Input: part model. Units: mm. Frame: model coordinates. Face numbers are marked on the shaded views. Coordinates: 2 decimals unless noted, no trailing zeros. Loops run counter-clockwise (first coordinate to the right, second up) from the corner with the lowest first, then second, coordinate; pieces in that order, holes last. Notation, with made-up numbers: (-15, 58) -> (43, 58) arc R30 cw to (43, 92) -> close; hole circle Ø4 at (-11.5, 48). An arc over 180 degrees is marked (long way). Answer as a JSON object with one key per item and string values.
from build123d import *

# Parameters (mm, degrees)
SKETCH_1_R          = 12.5
EXTRUDE_1_DEPTH     = 10
SKETCH_3_R          = 5
CUT_EXTRUDE_1_DEPTH = 11
CHAMFER_1_SIZE      = 7


with BuildPart() as part:
    # ｽｹｯﾁ1 → ﾎﾞｽ - 押し出し1 (new body)
    with BuildSketch(Plane.XY):
        Circle(SKETCH_1_R)
    extrude(amount=EXTRUDE_1_DEPTH)

    # ｽｹｯﾁ3 → ｶｯﾄ - 押し出し1 (cut, through all)
    with BuildSketch(Plane(origin=(0, 0, 0), x_dir=(-1, 0, 0), z_dir=(0, 0, -1))):
        Circle(SKETCH_3_R)
    extrude(amount=-CUT_EXTRUDE_1_DEPTH, mode=Mode.SUBTRACT)

    # 面取り1
    chamfer_1_edges = [part.edges().sort_by_distance(p)[0] for p in [
        (5, 0, 0),
    ]]
    chamfer(chamfer_1_edges, length=CHAMFER_1_SIZE)


solid = part.part
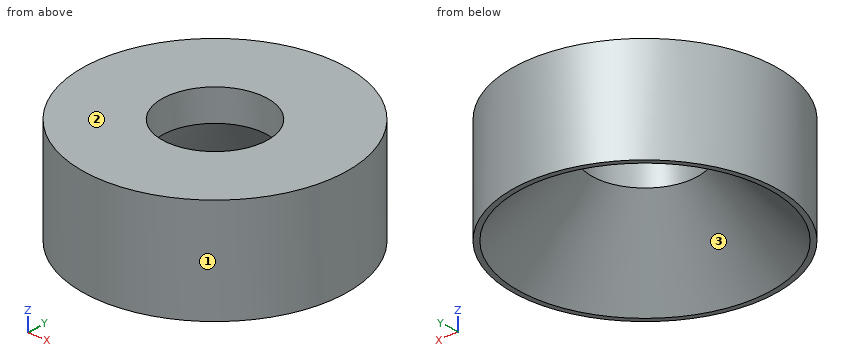
1. Section query A-A (x = 0). Return loops of the section in (y, z).
Reply:
{"outline": "(-12.5, 0) -> (-12, 0) -> (-5, 7) -> (-5, 10) -> (-12.5, 10) -> close; (5, 7) -> (12, 0) -> (12.5, 0) -> (12.5, 10) -> (5, 10) -> close"}
2. Section query B-B (z = 2.5). Return loops of the section in (x, y), plus the area to 3 significant figures.
Reply:
{"outline": "circle Ø25 at (0, 0); hole circle Ø19 at (0, 0)", "area": "207 mm2"}
3. Mould query, pull axis Y, two halves, no side actions, for the marked faces 1, 2 and 3. Classes: pulls with the +Y half, pulls with the -Y half, needs draft (parallel to the pull), parting line crosses it, or undercut.
Reply:
{"face 1": "parting line crosses it", "face 2": "needs draft", "face 3": "undercut"}
4. Pin query (flat end, axial travel): P1, Ø2, axis at x = 3, z = 4, coming from the -Y side; P2, Ø5, axis at x = -6, z = 8, coming from the +Y side; P3, Ø2, axis at x = -1, y = 9.5, coming from the -Z side. Return the tip coordinate at first contact, or that it passes through.
Reply:
{"P1": "stops at y = -12.34", "P2": "stops at y = 12", "P3": "stops at z = 1.45"}
5. Line query: line 1 along Y through (x, z) = (0, 9.2); line 2 along X through (y, z) = (-2.5, 1.75); line 3 along Y through (x, z) = (6, 3.75). Output: solid intervals per line, ascending.
Reply:
{"line 1": "y = -12.5 to -5, 5 to 12.5", "line 2": "x = -12.25 to -9.94, 9.94 to 12.25", "line 3": "y = -10.97 to -5.66, 5.66 to 10.97"}
6. Section query C-C (z = 9.5). Return loops of the section in (x, y), plus the area to 3 significant figures.
Reply:
{"outline": "circle Ø25 at (0, 0); hole circle Ø10 at (0, 0)", "area": "412 mm2"}
